Job drawing, mm, ordinate dimensions from the low corner. One solid piece. A direction names the side the tool comes from. Coordinates: 2 decimals unless noted, no trailing zeros. Order: outer loops, then holes, each group sorted by start corner. A loop starts at its lowest first (then second) coordinate and runs counter-clockwise, first axis right, second up. Notation, with made-up numbers: (6, -15.5) - (16, -15.5) arc R16 ccw to (16, -10.5) - close; hole circle Ø9 at (69.25, -32). An arc over 180 degrees is marked (long way). Return JSON: item names as keys, results as strings.
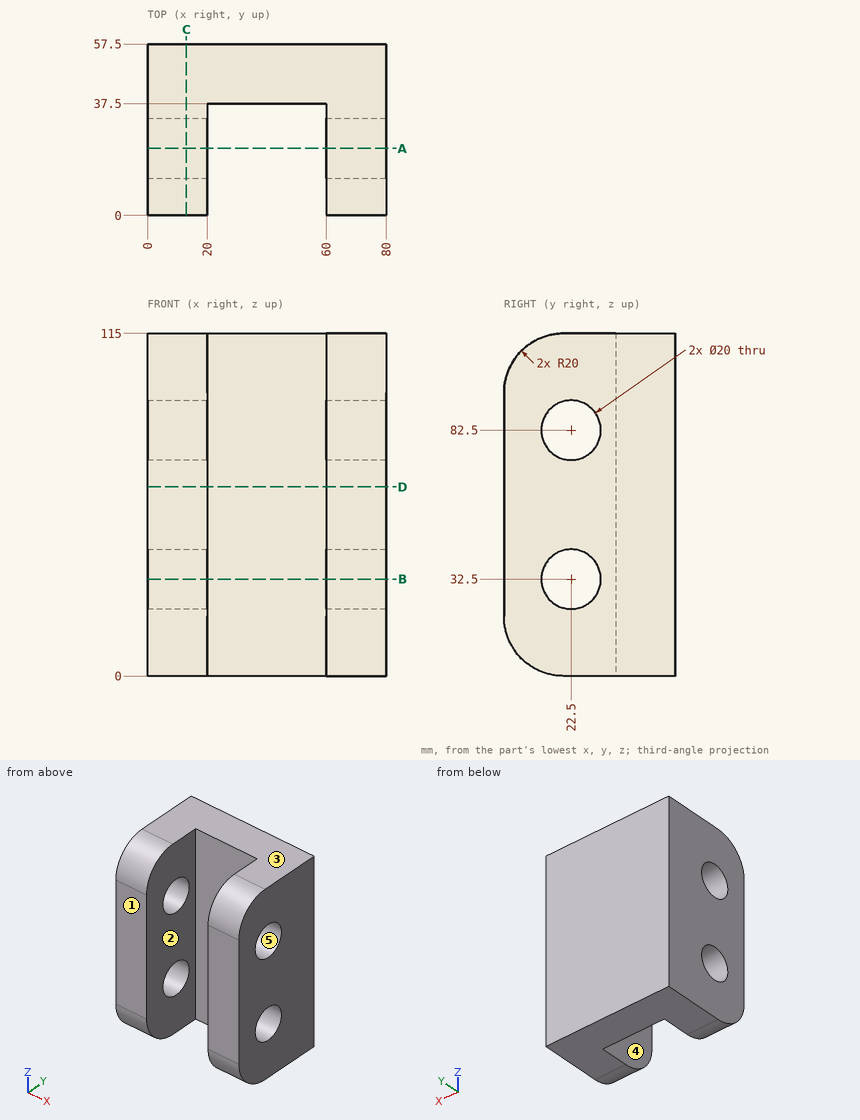
1. Probe L1, parallel to Z at x = 70, y = 22; L2, parallel to X at y = 36, z = 52.5; L3, parallel to Y at x = 30.5, z = 39. List the from-to ranges inside material, lowest first.
Check values:
{"L1": "0 to 22.51, 42.49 to 72.51, 92.49 to 115", "L2": "0 to 20, 60 to 80", "L3": "37.5 to 57.5"}
2. Drop flat-ended pins along their axis: pin 1 (1.5 mm diameter, centred on x = 68.5, y = 8.5, fed in from -Z); pin 2 (16 mm diameter, centred on y = 22.5, z = 82.5, fed in from -X); pin 3 (20 mm diameter, centred on x = 47.5, z = 55.5, fed in from -Y); pin 4 (2 mm diameter, centred on x = 65, y = 15.5, fed in from -Z). Give the stop position or say it passes through.
Check values:
{"pin 1": "z = 3.13", "pin 2": "through", "pin 3": "y = 37.5", "pin 4": "z = 0.31"}
3. Tool access for the marked faces 1 and 2: list every direction of +Z, -Z, +X, -X, +Y, -Y with a clear straight run to the whole face (end or side of a thin tool).
Check values:
{"face 1": "+Z, -Z, +X, -X, -Y", "face 2": "+Z, -Z, -Y"}
4. Cut at B-B on z = 32.5. Give the cut face in (x, y).
Check values:
{"outline": "(0, 0) - (20, 0) - (20, 12.5) - (0, 12.5) - close; (0, 32.5) - (20, 32.5) - (20, 37.5) - (60, 37.5) - (60, 32.5) - (80, 32.5) - (80, 57.5) - (0, 57.5) - close; (60, 0) - (80, 0) - (80, 12.5) - (60, 12.5) - close"}
5. Mould opens along Z. For the marked faces 3, 4 and 5 say: pulls with the +Z half, pulls with the -Z half, needs draft (parallel to the pull), parting line crosses it, or undercut.
Check values:
{"face 3": "pulls with the +Z half", "face 4": "needs draft", "face 5": "undercut"}
6. Cut at D-D on z = 63.5. Give the cut face in (x, y).
Check values:
{"outline": "(0, 0) - (20, 0) - (20, 37.5) - (60, 37.5) - (60, 0) - (80, 0) - (80, 57.5) - (0, 57.5) - close"}
7. Cut at C-C on x = 13. Give the cut face in (y, z).
Check values:
{"outline": "(0, 20) arc R20 ccw to (20, 0) - (57.5, 0) - (57.5, 115) - (20, 115) arc R20 ccw to (0, 95) - close; hole circle Ø20 at (22.5, 32.5); hole circle Ø20 at (22.5, 82.5)"}
8. Cut at A-A on y = 22.5. Give the cut face in (x, z), plus the area to 3 significant figures.
Check values:
{"outline": "(0, 0) - (20, 0) - (20, 22.5) - (0, 22.5) - close; (0, 42.5) - (20, 42.5) - (20, 72.5) - (0, 72.5) - close; (0, 92.5) - (20, 92.5) - (20, 115) - (0, 115) - close; (60, 0) - (80, 0) - (80, 22.5) - (60, 22.5) - close; (60, 42.5) - (80, 42.5) - (80, 72.5) - (60, 72.5) - close; (60, 92.5) - (80, 92.5) - (80, 115) - (60, 115) - close", "area": "3,000 mm²"}
